Geometry: see drawing. Coordinates: mm, zero at the bounding-box minimum. A direction names the side the tool comes from. Coordinates: 2 decimals unless noted, no trailing zeros. Write each loop counter-clockwise with the first axis right and the second up, starting at its lowest first coordinate (ties: lowest second). Pieces come first, ordered by that corner, then holes.
1) Line query: L1, parallel to Y at x = 6, z = 0.5; L2, parallel to Y at x = 4.5, z = 1.75 (1 decimal). Output: solid intervals per line, ascending.
2) Pin query (flat end, axial travel): pin 1 Ø1 at (x, z) = (9, 7.5) entering from +Y (1 decimal); pin 2 Ø3 at (y, z) = (7, 5) entering from +X; pin 3 Ø2 at (x, z) = (6, 5.5) entering from -Y. Return the tip coordinate at first contact, or that it passes through.
3) Set-up query: the marked faces 4 and 5. Return all of +Z, -Z, +X, -X, +Y, -Y with unobstructed straight access to the full face (end or side cutting, diameter ignored); none if empty.
4) Draft query along X for the marked faces 1, 2 and 3. Return one class per face: pulls with the +X half, pulls with the -X half, needs draft (parallel to the pull), parting line crosses it, or undercut.
5) Section query A-A (y = 6). Output: boundary loops of the cut face in (x, z).
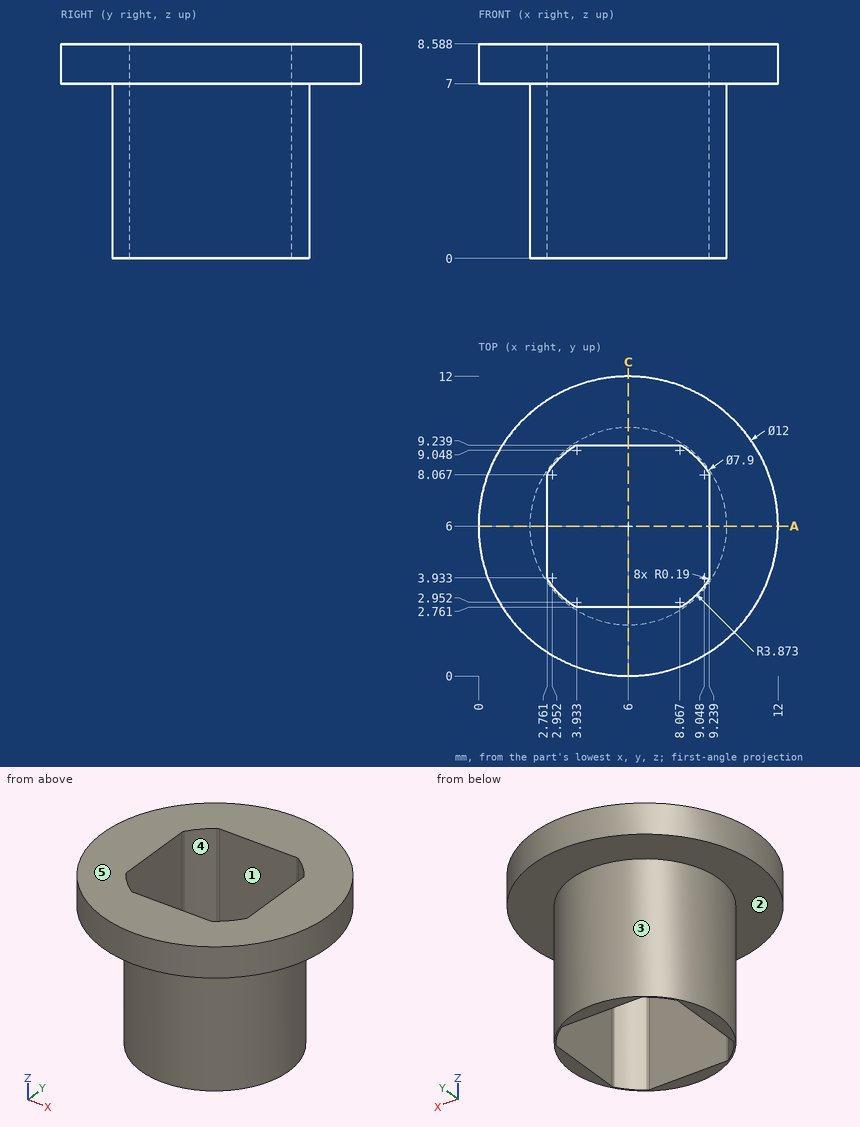
Answer:
1. L1: y = 2.05 to 2.76, 9.24 to 9.95
1. L2: y = 2.3 to 2.8, 9.2 to 9.7
2. pin 1: stops at y = 11.5
2. pin 2: stops at x = 9.95
2. pin 3: stops at y = 2.05
3. face 4: +Z, -Z
3. face 5: +Z, +X, -X, +Y, -Y
4. face 1: undercut
4. face 2: needs draft
4. face 3: parting line crosses it
5. outline: (0, 7) - (2.05, 7) - (2.05, 0) - (2.76, 0) - (2.76, 8.59) - (0, 8.59) - close; (9.24, 0) - (9.95, 0) - (9.95, 7) - (12, 7) - (12, 8.59) - (9.24, 8.59) - close
